Here's how the part is built. I have some questions about the finished solid (model axes, mm). A direction names the side the tool comes from. Coordinates: 2 decimals unless noted, no trailing zeros. Write each loop counter-clockwise with the first axis right and the second up, starting at its lowest first coordinate (ties: lowest second). Pieces come first, ordered by that corner, then holes.
(1) Imagine slicing it at A-A, the plane y = 0. List the corners of the cut face in (x, z) for me.
(2) Imagine slicing it at C-C, the plane x = 13. List the corners of the cut face in (y, z) for me, plus the area to 3 significant figures.
(3) Imagine slicing it at B-B, the plane x = -10. List the corners of the cut face in (y, z) for me.
(4) Imagine slicing it at D-D, the plane z = 0.65. State how many separate pieces and enclosed holes the cut face has, plus the area to 3 significant figures.
(5) Thinking about a two-plate mould opening in X: for faces 4 (the cylindrical face through (-18.334, -13.222, 0.501)), 5 (the cylindrical face through (8.414, 0.07, 0.501)), 6 (the flat face through (4, -3, 1.016)), 7 (the cylindrical face through (18.334, 13.222, 0.501)), which applies, released by +X, released by -X, zero draft, split by the parting line, or undercut?
(6) Please list where these lines run through material, in increasing order: probe 1 along Y at (x, z) = (0, 0.6); probe 2 along Y at (x, z) = (10, 0.8); probe 3 along X at (y, z) = (-10.5, 0.85).
(7) Which directions (+Z, -Z, +X, -X, +Y, -Y) give clear straight access to the entire face, cutting with the end or side of a thin tool? Please do faces 1 (the cylindrical face through (14.22, 20.24, 0.52)), 2 (the cylindrical face through (14.2, -20.22, 0.52)), 3 (the cylindrical face through (0.73, 8.59, 0.5)).
```python
from build123d import *

# Parameters (mm, degrees)
SKETCH1_R           = 22.6042
SKETCH1_R_2         = 1.5875
SKETCH1_R_3         = 1.3208
SKETCH1_R_4         = 4
BOSS_EXTRUDE2_DEPTH = 1.016
BOSS_EXTRUDE4_DEPTH = 1.016
CIRPATTERN1_COUNT   = 10


with BuildPart() as part:
    # Sketch1 → Boss-Extrude2 (new body)
    with BuildSketch(Plane.XY):
        Circle(SKETCH1_R)
        with Locations((0, 10)):
            Circle(SKETCH1_R_2, mode=Mode.SUBTRACT)
        with Locations((9.878281733, -9.878281733)):
            Circle(SKETCH1_R_3, mode=Mode.SUBTRACT)
        with Locations((9.878281733, 9.878281733)):
            Circle(SKETCH1_R_3, mode=Mode.SUBTRACT)
        with Locations((-9.878281733, -9.878281733)):
            Circle(SKETCH1_R_3, mode=Mode.SUBTRACT)
        with Locations((-9.878281733, 9.878281733)):
            Circle(SKETCH1_R_3, mode=Mode.SUBTRACT)
        Circle(SKETCH1_R_4, mode=Mode.SUBTRACT)
        with Locations((10, 0)):
            Circle(SKETCH1_R_2, mode=Mode.SUBTRACT)
        with Locations((0, -10)):
            Circle(SKETCH1_R_2, mode=Mode.SUBTRACT)
        with Locations((-10, 0)):
            Circle(SKETCH1_R_2, mode=Mode.SUBTRACT)
    extrude(amount=BOSS_EXTRUDE2_DEPTH)

    # Sketch2 → Boss-Extrude4 (add)
    with BuildSketch(Plane.XY.offset(1.016)):
        with BuildLine():
            ThreePointArc((0.499966183, 23.867964213), (0.39548978, 24.71817963), (0.088277099, 25.517805758))
            ThreePointArc((0.088277099, 25.517805758), (2.11e-07, 25.570824608), (-0.088276453, 25.517805384))
            ThreePointArc((-0.088276453, 25.517805384), (-0.395485603, 24.718178984), (-0.499958974, 23.867964213))
            ThreePointArc((-0.499958974, 23.867964213), (-0.860359014, 23.002073844), (-1.63911586, 22.479396033))
            ThreePointArc((-1.63911586, 22.479396033), (3.604e-06, 22.249732232), (1.639123068, 22.479396033))
            ThreePointArc((1.639123068, 22.479396033), (0.860366222, 23.002073844), (0.499966183, 23.867964213))
        make_face()
    boss_extrude4 = extrude(amount=-BOSS_EXTRUDE4_DEPTH)

    # CirPattern1: Boss-Extrude4 ×10 about axis
    cirpattern1_axis = Axis((0, 0, 0), (0, 0, 1))
    for i in range(1, CIRPATTERN1_COUNT):
        add(boss_extrude4.rotate(cirpattern1_axis, i * 360 / CIRPATTERN1_COUNT))


solid = part.part
```
Recorded:
1. outline: (-22.6, 0) - (-11.59, 0) - (-11.59, 1.02) - (-22.6, 1.02) - close; (-8.41, 0) - (-4, 0) - (-4, 1.02) - (-8.41, 1.02) - close; (4, 0) - (8.41, 0) - (8.41, 1.02) - (4, 1.02) - close; (11.59, 0) - (22.6, 0) - (22.6, 1.02) - (11.59, 1.02) - close
2. outline: (-19.17, 0) - (19.17, 0) - (19.17, 1.02) - (-19.17, 1.02) - close
2. area: 39.0 mm2
3. outline: (-20.27, 0) - (-11.19, 0) - (-11.19, 1.02) - (-20.27, 1.02) - close; (-8.56, 0) - (-1.59, 0) - (-1.59, 1.02) - (-8.56, 1.02) - close; (1.59, 0) - (8.56, 0) - (8.56, 1.02) - (1.59, 1.02) - close; (11.19, 0) - (20.27, 0) - (20.27, 1.02) - (11.19, 1.02) - close
4. separate pieces: 1
4. enclosed holes: 9
4. area: 1,530 mm2
5. face 4: released by -X
5. face 5: undercut
5. face 6: zero draft
5. face 7: released by +X
6. probe 1: y = -25.57 to -11.59, -8.41 to -4, 4 to 8.41, 11.59 to 25.57
6. probe 2: y = -20.27 to -11.19, -8.56 to -1.59, 1.59 to 8.56, 11.19 to 20.27
6. probe 3: x = -20.02 to -11.04, -8.71 to -1.51, 1.51 to 8.71, 11.04 to 20.02
7. face 1: +Z, -Z, +Y
7. face 2: +Z, -Z, -Y
7. face 3: +Z, -Z
